Autodesk Inventor part; units mm, degrees
ref_plane "YZ Plane" through (0, 0, 0) normal (1, 0, 0) x (0, 1, 0)
ref_plane "XZ Plane" through (0, 0, 0) normal (0, 1, 0) x (-1, 0, 0)
ref_plane "XY Plane" through (0, 0, 0) normal (0, 0, 1) x (1, 0, 0)
sketch "Sketch1" plane through (0, 0, 0) normal (0, 0, 1) x (1, 0, 0)
  line L0 (-52.5, 0) -> (52.5, 0)
  line L1 (0, -52.5) -> (0, 52.5)
  line L2 (-37.5, -37.5) -> (37.5, -37.5)
  line L3 (37.5, -37.5) -> (37.5, 37.5)
  line L4 (37.5, 37.5) -> (-37.5, 37.5)
  line L5 (-37.5, 37.5) -> (-37.5, -37.5)
  line L6 (-37.5, -37.5) -> (37.5, 37.5) construction
  line L7 (37.5, -37.5) -> (-37.5, 37.5) construction
  point P0 (0, 0)
  dimension "d0" = 75
  dimension "d1" = 75
extrude "Extrusion1" add sketch "Sketch1" along normal blind 3
sketch "Sketch2" plane through (0, 0, 3) normal (0, 0, 1) x (1, 0, 0)
  line L0 (37.5, -37.5) -> (37.5, 37.5)
  line L1 (37.5, 37.5) -> (-37.5, 37.5)
  line L2 (37.5, 17.5) -> (37.5, 27.5)
  line L3 (37.5, 27.5) -> (-37.5, 27.5)
  line L4 (-37.5, 27.5) -> (-37.5, 17.5)
  line L5 (-37.5, 17.5) -> (37.5, 17.5)
  point P0 (0, 0)
  dimension "d4" = 10
  dimension "d5" = 10
extrude "Extrusion2" add sketch "Sketch2" along normal blind 15
chamfer "Chamfer1" distance 2.5 angle 45 2 edges at (37.5, 22.5, 18) (-37.5, 22.5, 18)
sketch "Sketch3" plane through (0, 0, 18) normal (0, 0, 1) x (1, 0, 0)
  line L0 (-35, 17.5) -> (-35, 27.5)
  line L1 (35, 27.5) -> (35, 17.5)
  line L2 (-35, 22.5) -> (35, 22.5) construction
  circle A0 centre (-5, 22.5) radius 1.75
  circle A1 centre (-22.5, 22.5) radius 1.75
  line L3 (0, -52.5) -> (0, 52.5)
  circle A2 centre (22.5, 22.5) radius 1.75
  point P0 (0, 0)
  dimension "d11" = 45
  dimension "d12" = 17.5
  dimension "d13" = 5
  dimension "d14" = 3.5
extrude "Extrusion3" cut sketch "Sketch3" against normal through all
sketch "Sketch4" plane through (0, 0, 0) normal (0, 0, -1) x (-1, 0, 0)
  circle A0 centre (22.5, 22.5) radius 1.75
  circle A1 centre (5, 22.5) radius 1.75
  circle A2 centre (-22.5, 22.5) radius 1.75
  line L0 (37.5, -37.5) -> (-37.5, -37.5)
  line L1 (37.5, 37.5) -> (37.5, -37.5)
  line L2 (-37.5, 37.5) -> (37.5, 37.5)
  line L3 (-37.5, -37.5) -> (-37.5, 37.5)
  circle A3 centre (-22.5, 22.5) radius 3.25
  circle A4 centre (5, 22.5) radius 3.25
  circle A5 centre (22.5, 22.5) radius 3.25
  point P0 (0, 0)
  dimension "d17" = 6.5
properties part number "misc_hand_stand"
Read the model definition and answer for the solid it produces. Units are mm, in the model's axes. A direction names the side the tool comes from. Give positions to 0.01 mm unless a question says otherwise; leave off trailing zeros. Write each loop counter-clockwise with the first axis right and the second up, starting at its lowest first coordinate (ties: lowest second). Pieces come first, ordered by that corner, then holes. Notation, with made-up numbers: (18, 22) - (43, 22) arc R21 cw to (43, 42) - close; hole circle Ø2 at (87.5, 19.25). An arc over 180 degrees is marked (long way). Answer in a Markdown table with one row per item. Add a question column.
Item 1: Section C-C, the plane y = 22.5 is taken. Write down the section's boundary in (x, z).
Item 2: A tool of negligible diameter and unlimited length cuts with its end or side. For faces 1 (the face through (0, 23, 18)), 2 (the face through (-1, -10, 3)), 3 (the face through (1, 27.5, 10)), from which of +Z, -Z, +X, -X, +Y, -Y can it reach the whole face along a straight path? Write none if from no direction.
Item 3: Section B-B, the plane x = -5 is taken. Write down the section's boundary in (y, z).
Item 4: Find the intervals of material crossed by L1, parallel to Y at x = -5, z = 11.25; L2, parallel to Y at x = 29.5, z = 10; L3, parallel to Z at x = 0.5, y = 0, in increasing order.
Item 5: Determine the mould class of faces 4 (the face through (-1, -37.5, 1)), 5 (the face through (37.5, 8.2, 2.5)), 6 (the face through (-5.228, 24.235, 9.126)), 7 (the face through (21.21, 23.68, 9.13)) for opening direction X: pulls with the +X half, pulls with the -X half, needs draft (parallel to the pull), parting line crosses it, or undercut.
Item 6: Flat-ended cylindrical pins translate along their axes: P1, Ø10, axis at x = 16, y = 5, coming from the +Z side; P2, Ø8, axis at x = -22, z = 11, coming from the -Y side. Find the tip coordinate at first contact, or state that the pin passes through.
Item 7: Section A-A, the plane z = 8.75 is taken. Write down the section's boundary in (x, y), and give its area (3 significant figures).
Item 8: Section D-D, the plane x = 33.5 is taken. Write down the section's boundary in (y, z).
Recorded:
| question | item | result |
|---|---|---|
| 1 | outline | (-37.5, 0) - (-24.25, 0) - (-24.25, 18) - (-35, 18) - (-37.5, 15.5) - close; (-20.75, 0) - (-6.75, 0) - (-6.75, 18) - (-20.75, 18) - close; (-3.25, 0) - (20.75, 0) - (20.75, 18) - (-3.25, 18) - close; (24.25, 0) - (37.5, 0) - (37.5, 15.5) - (35, 18) - (24.25, 18) - close |
| 2 | face 1 | +Z, +X, -X, +Y, -Y |
| 2 | face 2 | +Z, +X, -X, -Y |
| 2 | face 3 | +Z, +X, -X, +Y |
| 3 | outline | (-37.5, 0) - (20.75, 0) - (20.75, 18) - (17.5, 18) - (17.5, 3) - (-37.5, 3) - close; (24.25, 0) - (37.5, 0) - (37.5, 3) - (27.5, 3) - (27.5, 18) - (24.25, 18) - close |
| 4 | L1 | y = 17.5 to 20.75, 24.25 to 27.5 |
| 4 | L2 | y = 17.5 to 27.5 |
| 4 | L3 | z = 0 to 3 |
| 5 | face 4 | needs draft |
| 5 | face 5 | pulls with the +X half |
| 5 | face 6 | undercut |
| 5 | face 7 | undercut |
| 6 | P1 | stops at z = 3 |
| 6 | P2 | stops at y = 17.5 |
| 7 | outline | (-37.5, 17.5) - (37.5, 17.5) - (37.5, 27.5) - (-37.5, 27.5) - close; hole circle Ø3.5 at (-22.5, 22.5); hole circle Ø3.5 at (-5, 22.5); hole circle Ø3.5 at (22.5, 22.5) |
| 7 | area | 721 mm2 |
| 8 | outline | (-37.5, 0) - (37.5, 0) - (37.5, 3) - (27.5, 3) - (27.5, 18) - (17.5, 18) - (17.5, 3) - (-37.5, 3) - close |
